Could you check a few things on this drawing? It's one solid part, dimensions in mm from its lowest x, y, z. A direction names the side the tool comes from. Coordinates: 2 decimals unless noted, no trailing zeros. Write each loop counter-clockwise with the first axis right and the second up, starting at its lowest first coordinate (ties: lowest second). Pieces come first, ordered by that corner, then holes. Notation, with made-up numbers: M 80,-8.5 L 112,-8.5 A29 ccw 112,29.5 Z; hole C 72.25,-3.5 d8. An arc over 180 degrees is marked long. Use a Markdown table: item, result.
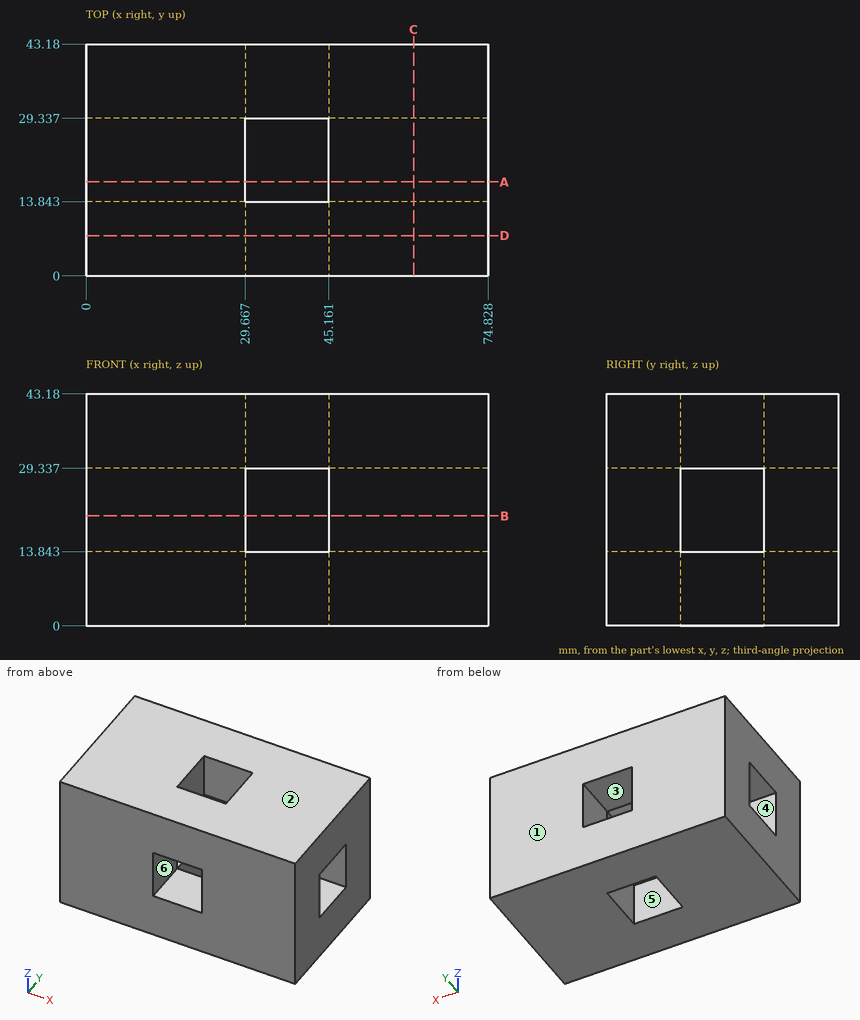
1. Suppose I cut it at D-D on y = 7.5. Write out the boundary of the cut face in (x, z).
Answers follow:
| item | result |
|---|---|
| outline | M 0,0 L 74.83,0 L 74.83,43.18 L 0,43.18 Z; hole M 29.67,13.84 L 45.16,13.84 L 45.16,29.34 L 29.67,29.34 Z |
2. Suppose I cut it at C-C on x = 61. Write out the boundary of the cut face in (y, z).
Answers follow:
| item | result |
|---|---|
| outline | M 0,0 L 43.18,0 L 43.18,43.18 L 0,43.18 Z; hole M 13.84,13.84 L 29.34,13.84 L 29.34,29.34 L 13.84,29.34 Z |
3. I need wall thicknesses on probe 1 along X at (y, z) = (26, 36.5); probe 2 along Z at (x, y) = (58.5, 28). Which ranges of each line are inside material? Lowest first, please.
Answers follow:
| item | result |
|---|---|
| probe 1 | x = 0 to 29.67, 45.16 to 74.83 |
| probe 2 | z = 0 to 13.84, 29.34 to 43.18 |
4. Will these pins go through, and if not, where does the flat tip stop? pin 1 Ø2 at (x, z) = (21, 26.5) entering from -Y; pin 2 Ø2 at (y, z) = (15.5, 17.5) entering from -X.
Answers follow:
| item | result |
|---|---|
| pin 1 | stops at y = 0 |
| pin 2 | passes through |
5. Suppose I cut it at A-A on y = 17.5. Write out the boundary of the cut face in (x, z), and give its area (3 significant figures).
Answers follow:
| item | result |
|---|---|
| outline | M 0,0 L 29.67,0 L 29.67,13.84 L 0,13.84 Z; M 0,29.34 L 29.67,29.34 L 29.67,43.18 L 0,43.18 Z; M 45.16,0 L 74.83,0 L 74.83,13.84 L 45.16,13.84 Z; M 45.16,29.34 L 74.83,29.34 L 74.83,43.18 L 45.16,43.18 Z |
| area | 1,640 mm2 |
6. We'd pull the mould along Z, two halves only. Please class the marked faces 1, 2 and 3: +Z half, -Z half, draft (parallel to the pull), parting line (faces both ways), or undercut.
Answers follow:
| item | result |
|---|---|
| face 1 | draft |
| face 2 | +Z half |
| face 3 | undercut |
7. Which directions (+Z, -Z, +X, -X, +Y, -Y) give clear straight access to the entire face, cutting with the end or side of a thin tool? Please do the marked faces 4, 5 and 6.
Answers follow:
| item | result |
|---|---|
| face 4 | +X, -X |
| face 5 | +Z, -Z |
| face 6 | +Y, -Y |
